Source: CAD feature listing. Evaluate the final solid. Frame: model axes, mm. Give positions to 0.01 mm unless a question says otherwise; leave off trailing zeros. Order: outer loops, then holes, each group sorted by start corner. A loop starts at its lowest first (then second) coordinate and runs counter-clockwise, first axis right, second up. Notation, with made-up numbers: M 36.5,89 L 51.5,89 A21 cw 51.5,113 Z; hole C 29.5,8 d11. An arc over 180 degrees is marked long. Answer as a JSON object with one key per item and string values. Group by question number.
1. Material intervals for L1, parallel to Y at x = 0, z = 305.5; L2, parallel to Y at x = 1.75, z = 126; L3, parallel to Y at x = -1.5, z = 181, sorted ascending. Write a range as [from, to].
2. Section query A-A (y = 0). Output: boundary loops of the cut face in (x, z), plus the area to 3 significant figures.
3. Pin query (flat end, axial travel): P1, Ø2, axis at y = 6, z = -119.5, coming from the +X side; P2, Ø4.5, axis at x = 0, y = 0, coming from the +Z side; P3, Ø1, axis at y = 4.5, z = 199, coming from the +X side. Return the tip coordinate at first contact, or that it passes through.
4. Section query B-B (z = -247). Output: boundary loops of the cut face in (x, y).
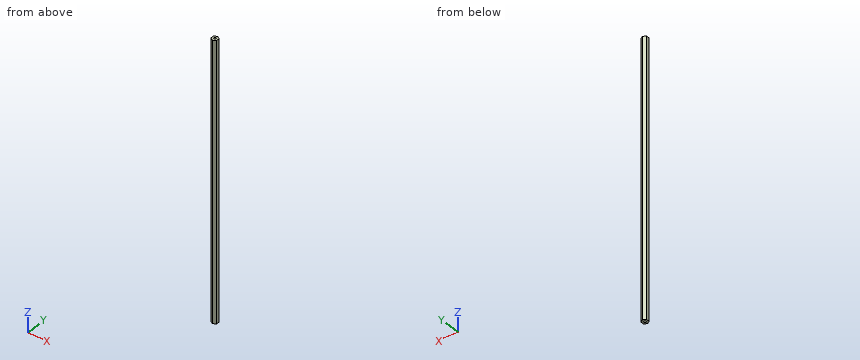
from build123d import *

# Parameters (mm, degrees)
BOSS_EXTRUDE1_DEPTH = 315.9125
SKETCH2_R           = 2.4892
CUT_EXTRUDE1_DEPTH  = 19.05


with BuildPart() as part:
    # Sketch1 → Boss-Extrude1 (new, symmetric)
    with BuildSketch(Plane.XY):
        Polygon((6.35, -3.666174209), (6.35, 3.666174209), (0, 7.332348419), (-6.35, 3.666174209), (-6.35, -3.666174209), (0, -7.332348419), align=None)
    extrude(amount=BOSS_EXTRUDE1_DEPTH, both=True)

    # Sketch2 → Cut-Extrude1 (cut)
    with BuildSketch(Plane.XY.offset(315.9125)):
        Circle(SKETCH2_R)
    cut_extrude1 = extrude(amount=-CUT_EXTRUDE1_DEPTH, mode=Mode.SUBTRACT)

    # Mirror1: Cut-Extrude1 across plane
    add(cut_extrude1.mirror(Plane.XY), mode=Mode.SUBTRACT)


solid = part.part
Answer sheet:
{
 "1": {"L1": "[-7.33, -2.49], [2.49, 7.33]", "L2": "[-6.32, 6.32]", "L3": "[-6.47, 6.47]"},
 "2": {"outline": "M -6.35,-315.91 L -2.49,-315.91 L -2.49,-296.86 L 2.49,-296.86 L 2.49,-315.91 L 6.35,-315.91 L 6.35,315.91 L 2.49,315.91 L 2.49,296.86 L -2.49,296.86 L -2.49,315.91 L -6.35,315.91 Z", "area": "7,830 mm^2"},
 "3": {"P1": "x = 4.04", "P2": "z = 296.86", "P3": "x = 5.77"},
 "4": {"outline": "M -6.35,-3.67 L 0,-7.33 L 6.35,-3.67 L 6.35,3.67 L 0,7.33 L -6.35,3.67 Z"}
}
